Part model, mm, in its own coordinate system. Face numbers are marked on the shaded views. A direction names the side the tool comes from. Coordinates: 2 decimals unless noted, no trailing zeros. Order: outer loops, then holes, each group sorted by start corner. A loop starts at its lowest first (then second) coordinate and runs counter-clockwise, first axis right, second up.
1) Wall check: L1, parallel to Y at x = -2.5, z = 21; L2, parallel to Z at x = -4.75, y = 5.75; L3, parallel to Y at x = -0.25, z = 11.75. Give the ranges that are in metal, low to high.
2) Cut at B-B (x = 1). List the corners of the cut face in (y, z).
3) Pin check, flat tips, straight feed: pin 1 Ø1.5 at (y, z) = (-4, 6.5) entering from -X; pin 2 Ø4 at (x, y) = (2, -0.5) entering from +Z; pin 3 Ø4 at (x, z) = (-1.5, 22) entering from -Y. Stop position of each tip, or through.
4) Cut at C-C (z = 3). List the corners of the cut face in (x, y), and give its area (3 significant figures).
5) Tool access for the marked faces 1, 2, 3 and 4: list every direction of +Z, -Z, +X, -X, +Y, -Y with a clear straight run to the whole face (end or side of a thin tool).
```python
from build123d import *

# Parameters (mm, degrees)
F0_R     = 6.35
F1_DEPTH = 20.32
F2_W     = 12.8309261054
F2_H     = 12.2810313478
F3_DEPTH = 5.08
F4_SIZE2 = 8.798808
F4_SIZE  = 5.07999


# Not quite as in the source:
# - a fillet or chamfer is up to 0.001 mm smaller than in the source, because OpenCascade refuses the exact size


with BuildPart() as f1:
    # F0 (on Top) → F1 (new body)
    with BuildSketch(Plane.XY):
        Circle(F0_R)
    extrude(amount=F1_DEPTH)

    # F2 (on face) → F3 (join)
    with BuildSketch(Plane.XY.offset(20.32)):
        Rectangle(F2_W, F2_H)
    extrude(amount=F3_DEPTH)

    # F4 (size 5.08 and 8.7988181024 in the source; OpenCascade refuses exactly that, so slightly less here)
    f4_edges = [f1.edges().sort_by_distance(p)[0] for p in [
        (6.415463, 0, 25.4),
    ]]
    f4_side = f1.faces().sort_by_distance((6.415463, 0, 22.86))[0]
    chamfer(f4_edges, length=F4_SIZE, length2=F4_SIZE2, reference=f4_side)


solid = f1.part
```
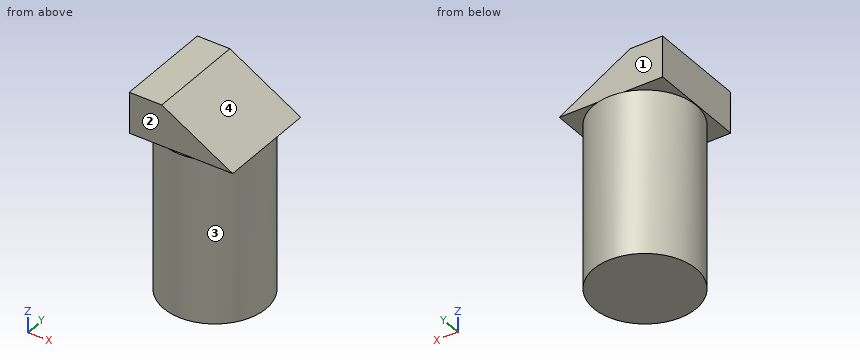
Geometry check:
1. L1: y = -6.14 to 6.14
1. L2: z = 20.32 to 25.4
1. L3: y = -6.35 to 6.35
2. outline: (-6.27, 0) - (6.27, 0) - (6.27, 20.32) - (6.14, 20.32) - (6.14, 23.45) - (-6.14, 23.45) - (-6.14, 20.32) - (-6.27, 20.32) - close
3. pin 1: stops at x = -5.46
3. pin 2: stops at z = 24.02
3. pin 3: stops at y = -6.34
4. outline: circle Ø12.7 at (0, 0)
4. area: 127 mm2
5. face 1: +Z, +X, -X, +Y
5. face 2: +Z, +X, -X, -Y
5. face 3: -Z
5. face 4: +Z, +X, +Y, -Y
